Read the model definition and answer for the solid it produces. Units are mm, in the model's axes. A direction names the side the tool comes from. Coordinates: 2 decimals unless noted, no trailing zeros. Loops run counter-clockwise (first coordinate to the right, second up) from the corner with the lowest first, then second, coordinate; pieces in that order, holes last. Notation, with made-up numbers: M -18,-13.5 L 41,-13.5 A13 ccw 41,0.5 Z; hole C -10,67 d8. An arc over 180 degrees is marked long. Put each result on its own line as item: value.
from build123d import *

# Parameters (mm, degrees)
ESQUISSE1_W             = 43.48
ESQUISSE1_H             = 160.19
BOSS_EXTRU_1_DEPTH      = 3
ESQUISSE2_R             = 4
BOSS_EXTRU_2_DEPTH      = 3
ENL_V_MAT_EXTRU_1_REACH = 104.065
ESQUISSE3_W             = 25.5
ESQUISSE3_H             = 14.4
CHANFREIN1_SIZE         = 3
CONG_1_R                = 5
ESQUISSE4_R             = 9
ENL_V_MAT_EXTRU_2_DEPTH = 2


# Some blends are built 0.0001 mm under size
with BuildPart() as part:
    # Esquisse1 → Boss.-Extru.1 (new body)
    with BuildSketch(Plane.XY):
        with BuildLine():
            Line((24.74, -69.15), (24.74, 93.04))
            ThreePointArc((24.74, 93.04), (24.154213562, 94.454213562), (22.74, 95.04))
            Line((22.74, 95.04), (-22.74, 95.04))
            ThreePointArc((-22.74, 95.04), (-24.154213562, 94.454213562), (-24.74, 93.04))
            Line((-24.74, 93.04), (-24.74, -69.15))
            ThreePointArc((-24.74, -69.15), (-24.154213562, -70.564213562), (-22.74, -71.15))
            Line((-22.74, -71.15), (22.74, -71.15))
            ThreePointArc((22.74, -71.15), (24.154213562, -70.564213562), (24.74, -69.15))
        make_face()
        with Locations((0, 11.945)):
            Rectangle(ESQUISSE1_W, ESQUISSE1_H, mode=Mode.SUBTRACT)
    extrude(amount=-BOSS_EXTRU_1_DEPTH)

    # Esquisse2 → Boss.-Extru.2 (add)
    with BuildSketch(Plane.XY):
        with BuildLine():
            Line((-22.74, -74.15), (22.74, -74.15))
            ThreePointArc((22.74, -74.15), (26.275533906, -72.685533906), (27.74, -69.15))
            Line((27.74, -69.15), (27.74, 93.04))
            ThreePointArc((27.74, 93.04), (26.275533906, 96.575533906), (22.74, 98.04))
            Line((22.74, 98.04), (-22.74, 98.04))
            ThreePointArc((-22.74, 98.04), (-26.275533906, 96.575533906), (-27.74, 93.04))
            Line((-27.74, 93.04), (-27.74, -69.15))
            ThreePointArc((-27.74, -69.15), (-26.275533906, -72.685533906), (-22.74, -74.15))
        make_face()
        with Locations((0.548, -9.9)):
            Circle(ESQUISSE2_R, mode=Mode.SUBTRACT)
    extrude(amount=BOSS_EXTRU_2_DEPTH)

    # Esquisse3 → Enlèv. mat.-Extru.1 (cut, up to next)
    with BuildSketch(Plane.XY.offset(3), mode=Mode.PRIVATE) as enl_v_mat_extru_1_sk1:
        with Locations((1.690390628, 18.008987034)):
            Rectangle(ESQUISSE3_W, ESQUISSE3_H)
    enl_v_mat_extru_1_tool1 = extrude(enl_v_mat_extru_1_sk1.sketch, amount=-ENL_V_MAT_EXTRU_1_REACH, mode=Mode.PRIVATE) & part.part
    add(enl_v_mat_extru_1_tool1.solids().sort_by_distance((1.690391, 18.008987, 3))[0], mode=Mode.SUBTRACT)

    # Chanfrein1
    chanfrein1_edges = [part.edges().sort_by_distance(p)[0] for p in [
        (14.440390628, 18.008987034, 3),
        (1.690390628, 10.808987034, 3),
        (-11.059609372, 18.008987034, 3),
        (1.690390628, 25.208987034, 3),
    ]]
    chamfer(chanfrein1_edges, length=CHANFREIN1_SIZE - 0.0001)  # a hair under: the kernel refuses the full size

    # Congé1
    # the kernel refuses this fillet: 5 mm, written as the material it takes off along each edge
    with BuildSketch(Plane(origin=(-27.74, 93.04, 3), x_dir=(1, 0, 0), z_dir=(0, -1, 0)), Plane(origin=(27.74, -69.15, 3), x_dir=(-1, 0, 0), z_dir=(0, 1, 0))) as cong_1_piece_1:
        with BuildLine():
            CenterArc((4.582575695, -5), CONG_1_R, 90, 66.421821522)
            Line((0, -3), (-0.091651514, -2.96))
            ThreePointArc((-0.091651514, -2.96), (-0.1, -1.5), (-0.1, 0))
            Line((-0.1, 0), (0, 0.1))
            Line((0, 0.1), (4.582575695, 0.1))
            Line((4.582575695, 0.1), (4.582575695, 0))
        make_face()
    extrude(amount=162.19, mode=Mode.SUBTRACT)
    with BuildSketch(Plane(origin=(-22.74, 93.04, 3), x_dir=(0, 1, 0), z_dir=(1, 0, 0))) as cong_1_piece_2:
        with BuildLine():
            CenterArc((0.417424305, -5), CONG_1_R, 23.578178478, 66.421821522)
            Line((5, -3), (5.091651514, -2.96))
            ThreePointArc((5.091651514, -2.96), (5.1, -1.5), (5.1, 0))
            Line((5.1, 0), (5, 0.1))
            Line((5, 0.1), (0.417424305, 0.1))
            Line((0.417424305, 0.1), (0.417424305, 0))
        make_face()
    revolve(axis=Axis((-22.74, 93.04, 3), (0, 0, 1)), revolution_arc=90, mode=Mode.SUBTRACT)
    with BuildSketch(Plane(origin=(22.74, 98.04, 3), x_dir=(0, -1, 0), z_dir=(-1, 0, 0)), Plane(origin=(-22.74, -74.15, 3), x_dir=(0, 1, 0), z_dir=(1, 0, 0))) as cong_1_piece_3:
        with BuildLine():
            CenterArc((4.582575695, -5), CONG_1_R, 90, 66.421821522)
            Line((0, -3), (-0.091651514, -2.96))
            ThreePointArc((-0.091651514, -2.96), (-0.1, -1.5), (-0.1, 0))
            Line((-0.1, 0), (0, 0.1))
            Line((0, 0.1), (4.582575695, 0.1))
            Line((4.582575695, 0.1), (4.582575695, 0))
        make_face()
    extrude(amount=45.48, mode=Mode.SUBTRACT)
    with BuildSketch(Plane(origin=(22.74, 93.04, 3), x_dir=(1, 0, 0), z_dir=(0, -1, 0))) as cong_1_piece_4:
        with BuildLine():
            CenterArc((0.417424305, -5), CONG_1_R, 23.578178478, 66.421821522)
            Line((5, -3), (5.091651514, -2.96))
            ThreePointArc((5.091651514, -2.96), (5.1, -1.5), (5.1, 0))
            Line((5.1, 0), (5, 0.1))
            Line((5, 0.1), (0.417424305, 0.1))
            Line((0.417424305, 0.1), (0.417424305, 0))
        make_face()
    revolve(axis=Axis((22.74, 93.04, 3), (0, 0, 1)), revolution_arc=90, mode=Mode.SUBTRACT)
    with BuildSketch(Plane(origin=(22.74, -69.15, 3), x_dir=(0, -1, 0), z_dir=(-1, 0, 0))) as cong_1_piece_5:
        with BuildLine():
            CenterArc((0.417424305, -5), CONG_1_R, 23.578178478, 66.421821522)
            Line((5, -3), (5.091651514, -2.96))
            ThreePointArc((5.091651514, -2.96), (5.1, -1.5), (5.1, 0))
            Line((5.1, 0), (5, 0.1))
            Line((5, 0.1), (0.417424305, 0.1))
            Line((0.417424305, 0.1), (0.417424305, 0))
        make_face()
    revolve(axis=Axis((22.74, -69.15, 3), (0, 0, 1)), revolution_arc=90, mode=Mode.SUBTRACT)
    with BuildSketch(Plane(origin=(-22.74, -69.15, 3), x_dir=(-1, 0, 0), z_dir=(0, 1, 0))) as cong_1_piece_6:
        with BuildLine():
            CenterArc((0.417424305, -5), CONG_1_R, 23.578178478, 66.421821522)
            Line((5, -3), (5.091651514, -2.96))
            ThreePointArc((5.091651514, -2.96), (5.1, -1.5), (5.1, 0))
            Line((5.1, 0), (5, 0.1))
            Line((5, 0.1), (0.417424305, 0.1))
            Line((0.417424305, 0.1), (0.417424305, 0))
        make_face()
    revolve(axis=Axis((-22.74, -69.15, 3), (0, 0, 1)), revolution_arc=90, mode=Mode.SUBTRACT)

    # Esquisse4 → Enlèv. mat.-Extru.2 (cut)
    with BuildSketch(Plane.XY.offset(3)):
        with Locations((0.548, -9.9)):
            Circle(ESQUISSE4_R)
    extrude(amount=-ENL_V_MAT_EXTRU_2_DEPTH, mode=Mode.SUBTRACT)


solid = part.part
1) Find section D-D, the plane y = 69. Write down the section's boundary in (x, z).
Answer list:
outline: M -27.74,0 L -24.74,0 L -24.74,-3 L -21.74,-3 L -21.74,0 L 21.74,0 L 21.74,-3 L 24.74,-3 L 24.74,0 L 27.74,0 A5 ccw 23.16,3 L -23.16,3 A5 ccw Z
2) Which of the six approach directions +Z, -Z, +X, -X, +Y, -Y give full straight-line access (tool end or side, diameter ignored) to faces 1 (the flat face through (21.74, 11, -1)), 2 (the cylindrical face through (-6.59, -15.38, 2.01)), 3 (the flat face through (0, -71.15, -1))?
Answer list:
face 1: -Z
face 2: +Z
face 3: -Z, +X, -X, -Y
3) Find section C-C, the plane y = -9.9. Write down the section's boundary in (x, z).
Answer list:
outline: M -27.74,0 L -24.74,0 L -24.74,-3 L -21.74,-3 L -21.74,0 L -3.45,0 L -3.45,1 L -8.45,1 L -8.45,3 L -23.16,3 A5 ccw Z; M 4.55,0 L 21.74,0 L 21.74,-3 L 24.74,-3 L 24.74,0 L 27.74,0 A5 ccw 23.16,3 L 9.55,3 L 9.55,1 L 4.55,1 Z
4) Given pin 1 Ø11 at (x, y) = (0.548, -9.9) entering from -Z; pin 2 Ø1.5 at (y, z) = (3.5, -1.5) entering from -X; pin 3 Ø0.9 at (x, z) = (-4.5, -2) entering from -Y, each flat-ended and moving along its own axis, determine where each tip first touches the part or whether it passes through.
Answer list:
pin 1: stops at z = 0
pin 2: stops at x = -24.74
pin 3: stops at y = -71.15
5) Find section B-B, the plane z = -1.15. Write down the section's boundary in (x, y).
Answer list:
outline: M -24.74,-69.15 A2 ccw -22.74,-71.15 L 22.74,-71.15 A2 ccw 24.74,-69.15 L 24.74,93.04 A2 ccw 22.74,95.04 L -22.74,95.04 A2 ccw -24.74,93.04 Z; hole M -21.74,-68.15 L 21.74,-68.15 L 21.74,92.04 L -21.74,92.04 Z
6) Determine the mould class of faces 4 (the cylindrical face through (0.318, 96.162, 2.205)), 5 (the flat face through (0, -68.15, -1)), 6 (the flat face through (-24.74, 13, -1)) for opening direction X: released by +X, released by -X, zero draft, split by the parting line, or undercut.
Answer list:
face 4: zero draft
face 5: undercut
face 6: released by -X
7) Straight lines are drawn through the part: line 1 (X direction, y = -14, z = -1); line 2 (Y direction, x = -6, z = -0.3); line 3 (Z direction, x = 7, y = -13). For each, find the intervals that lie inside material, in ascending order. Write a range as [from, to].
Answer list:
line 1: x = [-24.74, -21.74], [21.74, 24.74]
line 2: y = [-71.15, -68.15], [92.04, 95.04]
line 3: z = [0, 1]
